CAD build for the part. Positions are in the model's coordinates, mm. A direction names the side the tool comes from. Round coordinates to 2 decimals unless told otherwise and drop trailing zeros. Write each loop counter-clockwise with the first axis right and the second up, starting at its lowest first coordinate (ties: lowest second). Pieces come first, ordered by that corner, then holes. Notation, with made-up numbers: (-9.5, -38) - (9.5, -38) arc R25 ccw to (9.5, -2) - close; hole circle Ø9 at (61, 89.5). An arc over 180 degrees is marked (long way). Use one line per item in the form item = value. Start each with the question number.
Item 1: Pull direction Z, two halves, no side cores. Call faces 4 (the cylindrical face through (-1.5, 169.86, 14.77)), 5 (the flat face through (3, 180, 4)), 6 (the flat face through (-3, 2, 20)): +Z half, -Z half, draft (parallel to the pull), parting line (faces both ways), or undercut.
Item 2: Tool access for faces 1 (the flat face through (180, -160, 10)), 2 (the flat face through (-200, 2, 10)), 3 (the flat face through (0, 160, 10)): list every direction of +Z, -Z, +X, -X, +Y, -Y with a clear straight run to the whole face (end or side of a thin tool).
Item 3: Band-saw the part on A-A, the plane x = 180. List the corners of the cut face in (y, z).
Item 4: Drill centre lines: L1, parallel to X at y = -172.75, z = 10; L2, parallel to Z at x = -180, y = 169.75; L3, parallel to Y at x = -133.5, z = 1. Where is each one in solid material? Low to high.
Item 5: Pin check, flat tips, straight feed: pin 1 (5 mm diameter, centred on x = -1.5, z = 8.5, fed in from -Y); pin 2 (5 mm diameter, centred on x = 1, z = 10.5, fed in from +Y). Stop position of each tip, or through.
Solid Edge part; units mm, degrees
sketch "Sketch1" plane through (0, 0, 0) normal (0, 0, 1) x (1, 0, 0)
  line L0 (-200, -180) -> (200, -180)
  line L1 (200, -180) -> (200, 180)
  line L2 (200, 180) -> (-200, 180)
  line L3 (-200, 180) -> (-200, -180)
extrude "Protrusion1" add sketch "Sketch1" along normal blind 20
hole "Hole_1" at (-180, 180, 10) direction (0, -1, 0) diameter 10 depth 20
hole "Hole1" at (0, 180, 10) direction (0, -1, 0) diameter 10 depth 20
hole "Hole2" at (180, 180, 10) direction (0, -1, 0) diameter 10 depth 20
mirror "Mirror1" about plane through (0, 0, 0) normal (0, -1, 0) of "Hole_1", "Hole1", "Hole2"
fillet "Round_1" radius 1.5 12 edges at (0, -180, 20) (200, 0, 20) (0, 180, 20) (-200, 0, 20) (200, 180, 10) (200, -180, 10) (-200, 180, 10) (-200, -180, 10) (0, -180, 0) (-200, 0, 0) (200, 0, 0) (0, 180, 0)
properties material "Wood, Oak"
Determined:
q1.face_4 = undercut
q1.face_5 = draft
q1.face_6 = +Z half
q2.face_1 = -Y
q2.face_2 = +Z, -Z, -X, +Y, -Y
q2.face_3 = +Y
q3.outline = (-180, 1.5) arc R1.5 ccw to (-178.5, 0) - (178.5, 0) arc R1.5 ccw to (180, 1.5) - (180, 5) - (160, 5) - (160, 15) - (180, 15) - (180, 18.5) arc R1.5 ccw to (178.5, 20) - (-178.5, 20) arc R1.5 ccw to (-180, 18.5) - (-180, 15) - (-160, 15) - (-160, 5) - (-180, 5) - close
q4.L1 = -200 to -185, -175 to -5, 5 to 175, 185 to 200
q4.L2 = 0 to 5, 15 to 20
q4.L3 = -179.91 to 179.91
q5.pin_1 = -160
q5.pin_2 = 160
